from build123d import *

# Parameters (mm, degrees)
SKETCH1_R           = 9
BOSS_EXTRUDE1_DEPTH = 1.75
SKETCH2_R           = 1.5875
SKETCH2_W           = 4.7
SKETCH2_H           = 4.7
CUT_EXTRUDE1_DEPTH  = 2.75


with BuildPart() as part:
    # Sketch1 → Boss-Extrude1 (new body)
    with BuildSketch(Plane.XY):
        Circle(SKETCH1_R)
    extrude(amount=BOSS_EXTRUDE1_DEPTH)

    # Sketch2 → Cut-Extrude1 (cut, through all)
    with BuildSketch(Plane.XY.offset(1.75)):
        with Locations((0, 5.25)):
            Circle(SKETCH2_R)
        Rectangle(SKETCH2_W, SKETCH2_H)
    extrude(amount=-CUT_EXTRUDE1_DEPTH, mode=Mode.SUBTRACT)


solid = part.part
Source: CAD feature listing. Evaluate the final solid. Frame: model axes, mm. A direction names the side the tool comes from. Give positions to 0.01 mm unless a question says otherwise; leave off trailing zeros. Write each loop counter-clockwise with the first axis right and the second up, starting at its lowest first coordinate (ties: lowest second). Pieces come first, ordered by that corner, then holes. Notation, with made-up numbers: (10, 19.5) -> (38, 19.5) arc R14 cw to (38, 43.5) -> close; hole circle Ø4 at (88.5, 11.5). An arc over 180 degrees is marked (long way). Return JSON: item names as keys, results as strings. Group by question number.
1. Access query for faces 4 (the face through (0, -4, 1.75)), 5 (the face through (0, -2.35, 1)). Directions: +Z, -Z, +X, -X, +Y, -Y. A direction counts if a zero-diameter tool reaches every point of the face in a straight line with its end or side. Return the directions, or none.
2. Section C-C, the plane z = 1. Count the separate pieces of the cut face and the enclosed holes in it, then the cut area to 3 significant figures.
3. Pin query (flat end, axial travel): pin 1 Ø1 at (y, z) = (-3, 1) entering from -X; pin 2 Ø6 at (x, y) = (-4, -3) entering from -Z. Return the tip coordinate at first contact, or that it passes through.
4. Section D-D, the plane y = 5.25. Output: boundary loops of the cut face in (x, z), then the cut area to 3 significant figures.
5. Material intervals for line 1 (Y direction, x = 0, z = 1.1); line 2 (Y direction, x = -2, z = 0.3); line 3 (X direction, y = 0.5, z = 1.1), sorted ascending. Write a range as from..to.
6. Section B-B, the plane x = 0. Output: boundary loops of the cut face in (y, z).
7. Section A-A, the plane y = 0. Output: boundary loops of the cut face in (x, z).
8. Mould query, pull axis X, two halves, no side actions, for faces 1 (the face through (0, 2.35, 1)), 2 (the face through (-1.172, 8.923, 0.863)), 3 (the face through (0, -4, 0)). Classes: +X half, -X half, draft (parallel to the pull), parting line (faces both ways), or undercut.
Determined:
{
 "1": {"face 4": "+Z, +X, -X, +Y, -Y", "face 5": "+Z, -Z"},
 "2": {"separate pieces": "1", "enclosed holes": "2", "area": "224 mm2"},
 "3": {"pin 1": "stops at x = -8.65", "pin 2": "stops at z = 0"},
 "4": {"outline": "(-7.31, 0) -> (-1.59, 0) -> (-1.59, 1.75) -> (-7.31, 1.75) -> close; (1.59, 0) -> (7.31, 0) -> (7.31, 1.75) -> (1.59, 1.75) -> close", "area": "20.0 mm2"},
 "5": {"line 1": "y = -9..-2.35, 2.35..3.66, 6.84..9", "line 2": "y = -8.77..-2.35, 2.35..8.77", "line 3": "x = -8.99..-2.35, 2.35..8.99"},
 "6": {"outline": "(-9, 0) -> (-2.35, 0) -> (-2.35, 1.75) -> (-9, 1.75) -> close; (2.35, 0) -> (3.66, 0) -> (3.66, 1.75) -> (2.35, 1.75) -> close; (6.84, 0) -> (9, 0) -> (9, 1.75) -> (6.84, 1.75) -> close"},
 "7": {"outline": "(-9, 0) -> (-2.35, 0) -> (-2.35, 1.75) -> (-9, 1.75) -> close; (2.35, 0) -> (9, 0) -> (9, 1.75) -> (2.35, 1.75) -> close"},
 "8": {"face 1": "undercut", "face 2": "parting line", "face 3": "draft"}
}
